```python
from build123d import *

# Parameters (mm, degrees)
F0_W     = 1524
F0_H     = 711.2
F1_DEPTH = 25.4
F2_W     = 19.05
F2_H     = 355.6
F3_DEPTH = 90.4875
F4_W     = 1524
F4_H     = 355.6
F5_DEPTH = 19.05


with BuildPart() as f1:
    # F0 (on Top) → F1 (new body)
    with BuildSketch(Plane.XY):
        with Locations((762, 355.6)):
            Rectangle(F0_W, F0_H)
    extrude(amount=F1_DEPTH)

    # F2 (on face) → F3 (join)
    with BuildSketch(Plane.XY.offset(25.4)):
        with Locations((9.525, 533.4)):
            Rectangle(F2_W, F2_H)
        with Locations((511.175, 533.4)):
            Rectangle(F2_W, F2_H)
        with Locations((1012.825, 533.4)):
            Rectangle(F2_W, F2_H)
        with Locations((1514.475, 533.4)):
            Rectangle(F2_W, F2_H)
    extrude(amount=F3_DEPTH)

    # F4 (on face) → F5 (join)
    with BuildSketch(Plane.XY.offset(115.8875)):
        with Locations((762, 533.4)):
            Rectangle(F4_W, F4_H)
    extrude(amount=F5_DEPTH)


solid = f1.part
```
Here's how the part is built. I have some questions about the finished solid (model axes, mm). A direction names the side the tool comes from. Give positions to 0.01 mm unless a question says otherwise; leave off trailing zeros. Write each loop counter-clockwise with the first axis right and the second up, starting at its lowest first coordinate (ties: lowest second). Pieces come first, ordered by that corner, then holes.
(1) Will this pin go through, and if not, where does the flat tip stop? pin 1 (10 mm diameter, centred on x = 671, z = 19, fed in from -Y).
Output values:
pin 1: stops at y = 0
(2) Imagine slicing it at C-C, the plane y = 537. Write out the boundary of the cut face in (x, z).
Output values:
outline: (0, 0) - (1524, 0) - (1524, 134.94) - (0, 134.94) - close; hole (19.05, 25.4) - (501.65, 25.4) - (501.65, 115.89) - (19.05, 115.89) - close; hole (520.7, 25.4) - (1003.3, 25.4) - (1003.3, 115.89) - (520.7, 115.89) - close; hole (1022.35, 25.4) - (1504.95, 25.4) - (1504.95, 115.89) - (1022.35, 115.89) - close
(3) Imagine slicing it at B-B, the plane z = 76.5. Write out the boundary of the cut face in (x, y), and give its area (3 significant figures).
Output values:
outline: (0, 355.6) - (19.05, 355.6) - (19.05, 711.2) - (0, 711.2) - close; (501.65, 355.6) - (520.7, 355.6) - (520.7, 711.2) - (501.65, 711.2) - close; (1003.3, 355.6) - (1022.35, 355.6) - (1022.35, 711.2) - (1003.3, 711.2) - close; (1504.95, 355.6) - (1524, 355.6) - (1524, 711.2) - (1504.95, 711.2) - close
area: 27,100 mm2
(4) Imagine slicing it at A-A, the plane x = 1233. Write out the boundary of the cut face in (y, z), and give its area (3 significant figures).
Output values:
outline: (0, 0) - (711.2, 0) - (711.2, 25.4) - (0, 25.4) - close; (355.6, 115.89) - (711.2, 115.89) - (711.2, 134.94) - (355.6, 134.94) - close
area: 24,800 mm2
(5) Imagine slicing it at D-D, the plane y = 173. Write out the boundary of the cut face in (x, z), and give its area (3 significant figures).
Output values:
outline: (0, 0) - (1524, 0) - (1524, 25.4) - (0, 25.4) - close
area: 38,700 mm2
(6) Thinking about a two-plate mould opening in X: for faces 1 (the face through (1524, 509, 52)), 2 (the face through (751, 361, 25.4)), 3 (the face through (257, 536, 115.888)), 4 (the face through (751, 536, 134.938)), which applies, pulls with the +X half, pulls with the -X half, needs draft (parallel to the pull), parting line crosses it, or undercut?
Output values:
face 1: pulls with the +X half
face 2: undercut
face 3: undercut
face 4: needs draft
(7) On a 3-axis mill with a long thin cutter (end or side, diameter ignored), from which of +Z, -Z, +X, -X, +Y, -Y can I reach the whole of each face in a straight line? I mean faces 5 (the face through (751, 0, 13)), 6 (the face through (758, 355.6, 125)), 7 (the face through (520.7, 531, 70)). Say none if no direction works.
Output values:
face 5: +Z, -Z, +X, -X, -Y
face 6: +Z, +X, -X, -Y
face 7: +Y, -Y
(8) If I drill on L1, parallel to X at y = 525, z = 45; L2, parallel to Z at x = 1212, y = 593; L3, parallel to Y at x = 677.5, z = 127, over which ranges is the centre line in solid material (lowest first)?
Output values:
L1: x = 0 to 19.05, 501.65 to 520.7, 1003.3 to 1022.35, 1504.95 to 1524
L2: z = 0 to 25.4, 115.89 to 134.94
L3: y = 355.6 to 711.2
